For this review, take the finished solid that the model builds, in its own axes (mm). Face numbers are marked on the shaded views. A direction names the side the tool comes from. Round coordinates to 2 decimals unless told otherwise and drop trailing zeros. Loops run counter-clockwise (first coordinate to the right, second up) from the corner with the lowest first, then second, coordinate; pieces in that order, holes last. Notation, with made-up numbers: (19.5, -15) -> (40.5, -15) arc R14 ccw to (40.5, 8) -> close; hole circle Ø9 at (-3.5, -3). An arc over 180 degrees is marked (long way). Write each question's results on one line, items separated by ' | '.
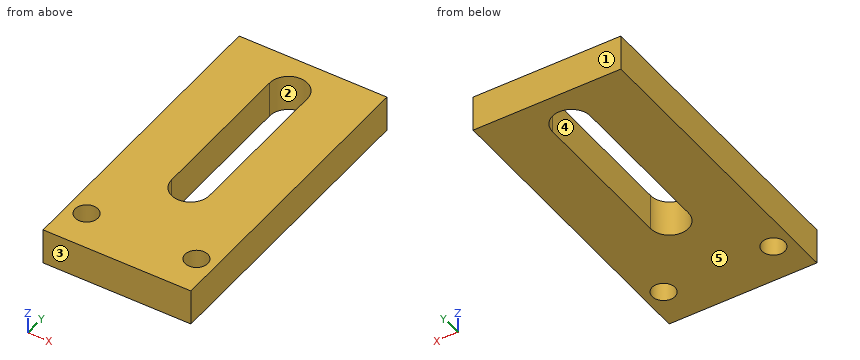
```python
from build123d import *

# Parameters (mm, degrees)
SKETCH1_4_R         = 1.5
BOSS_EXTRUDE3_DEPTH = 4.7625


with BuildPart() as part:
    # Sketch1_4 → Boss-Extrude3 (new body)
    # profile 1 of 5: a face of its own
    with BuildSketch(Plane.XY):
        with BuildLine():
            Line((0, 40), (0, 10))
            Line((0, 10), (7.25, 10))
            Line((7.25, 10), (7.25, 15.000000022))
            Line((7.25, 15.000000022), (7.25, 19.999999992))
            Line((7.25, 19.999999992), (7.25, 30.000000008))
            Line((7.25, 30.000000008), (7.25, 35))
            ThreePointArc((7.25, 35), (9.75, 37.5), (12.25, 35))
            Line((12.25, 35), (12.25, 30))
            Line((12.25, 30), (12.25, 20))
            Line((12.25, 20), (12.25, 15))
            Line((12.25, 15), (12.25, 10))
            Line((12.25, 10), (19.5, 10))
            Line((19.5, 10), (19.5, 40))
            Line((19.5, 40), (0, 40))
        make_face()
    # profile 2 of 5: a face of its own
    with BuildSketch(Plane.XY):
        with BuildLine():
            Line((0, 10), (0, 0))
            Line((0, 0), (19.5, 0))
            Line((19.5, 0), (19.5, 10))
            Line((19.5, 10), (12.25, 10))
            Line((12.25, 10), (12.25, 5))
            ThreePointArc((12.25, 5), (9.75, 2.5), (7.25, 5))
            Line((7.25, 5), (7.25, 10))
            Line((7.25, 10), (0, 10))
        make_face()
        with Locations(Location((2.5, 5, 0), (0, 0, 180))):
            Circle(SKETCH1_4_R, mode=Mode.SUBTRACT)
        with Locations(Location((17, 5, 0), (0, 0, 180))):
            Circle(SKETCH1_4_R, mode=Mode.SUBTRACT)
    # profile 3 of 5: a face of its own
    with BuildSketch(Plane.XY):
        with BuildLine():
            ThreePointArc((12.25, 5), (9.75, 7.5), (7.25, 5))
            ThreePointArc((7.25, 5), (9.75, 2.5), (12.25, 5))
        make_face()
    # profile 4 of 5: a face of its own
    with BuildSketch(Plane.XY):
        with BuildLine():
            Line((12.25, 10), (7.25, 10))
            Line((7.25, 10), (7.25, 5))
            ThreePointArc((7.25, 5), (9.75, 7.5), (12.25, 5))
            Line((12.25, 5), (12.25, 10))
        make_face()
    # profile 5 of 5: a face of its own
    with BuildSketch(Plane.XY):
        with BuildLine():
            Line((7.25, 15.000000022), (7.25, 10))
            Line((7.25, 10), (12.25, 10))
            Line((12.25, 10), (12.25, 15))
            ThreePointArc((12.25, 15), (9.749999989, 12.5), (7.25, 15.000000022))
        make_face()
    extrude(amount=BOSS_EXTRUDE3_DEPTH)


solid = part.part
```
1. To check wall thickness, follow probe 1 along X at (y, z) = (5, 3.75); probe 2 along Y at (x, z) = (2.5, 2.4); probe 3 along X at (y, z) = (33.5, 4.45). State the ranges of each line that lie inside material, in increasing order.
Values found:
probe 1: x = 0 to 1, 4 to 15.5, 18.5 to 19.5 | probe 2: y = 0 to 3.5, 6.5 to 40 | probe 3: x = 0 to 7.25, 12.25 to 19.5
2. Consider section A-A (y = 13). State the section outline as (x, z) points.
Values found:
outline: (0, 0) -> (8.25, 0) -> (8.25, 4.76) -> (0, 4.76) -> close; (11.25, 0) -> (19.5, 0) -> (19.5, 4.76) -> (11.25, 4.76) -> close
3. Tool access review of the marked faces 1 and 2: name each direction out of +Z, -Z, +X, -X, +Y, -Y from which nothing blocks a thin tool from reaching the whole face with its end or side.
Values found:
face 1: +Z, -Z, +X, -X, +Y | face 2: +Z, -Z
4. Consider section B-B (x = 17). State the section outline as (y, z) points, plus the area to 3 significant figures.
Values found:
outline: (0, 0) -> (3.5, 0) -> (3.5, 4.76) -> (0, 4.76) -> close; (6.5, 0) -> (40, 0) -> (40, 4.76) -> (6.5, 4.76) -> close | area: 176 mm2
5. Draft analysis for pull direction Y (two halves, no side actions). For the marked faces 3, 4 and 5, state which applies: released by +Y, released by -Y, zero draft, split by the parting line, or undercut.
Values found:
face 3: released by -Y | face 4: undercut | face 5: zero draft
6. Consider section C-C (z = 1.35). State the section outline as (x, y) points, plus the area to 3 significant figures.
Values found:
outline: (0, 0) -> (19.5, 0) -> (19.5, 40) -> (0, 40) -> close; hole circle Ø3 at (2.5, 5); hole (7.25, 15) arc R2.5 ccw to (12.25, 15) -> (12.25, 35) arc R2.5 ccw to (7.25, 35) -> close; hole circle Ø3 at (17, 5) | area: 646 mm2
7. Consider section D-D (y = 5). State the section outline as (x, z) points.
Values found:
outline: (0, 0) -> (1, 0) -> (1, 4.76) -> (0, 4.76) -> close; (4, 0) -> (15.5, 0) -> (15.5, 4.76) -> (4, 4.76) -> close; (18.5, 0) -> (19.5, 0) -> (19.5, 4.76) -> (18.5, 4.76) -> close
